```python
from build123d import *

# Parameters (mm, degrees)
F1_DEPTH = 40
F0_W     = 0.5
F0_H     = 12
F0_W_2   = 11.5
F0_W_3   = 12
F0_H_2   = 0.5
F0_H_3   = 14.25
F2_DEPTH = 5
F3_SIZE  = 2
F5_DEPTH = 0.5


with BuildPart() as f1:
    # F0 (on Top) → F1 (new body)
    with BuildSketch(Plane.XY):
        Polygon((17.2627416998, 5.4343145751), (15, 3.1715728753), (15, -3.1715728753), (17.2627416998, -5.4343145751), (17.2627416998, -0.5656854249), (17.2627416998, 0.5656854249), align=None)
        Polygon((-15, 29.1715728753), (-15, 4.1715728753), (-12.1715728752, 7), (-12.1715728752, 0), (-12.1715728752, -7), (-15, -4.1715728753), (-15, -29.1715728753), (15, -29.1715728753), (15, -3.1715728753), (15, 3.1715728753), (15, 29.1715728753), align=None)
        Polygon((-10.4999961331, 14.999999851), (-10.4999961331, 26.999999851), (1.5000038669, 26.999999851), (2.0000038669, 26.999999851), (13.5000038669, 26.999999851), (13.5000038669, 14.999999851), (13.5000038669, 14.499999851), (13.5000038669, 0.249999851), (13.5000038669, -0.250000149), (13.5000038669, -14.500000149), (13.5000038669, -15.000000149), (13.5000038669, -27.000000149), (2.0000038669, -27.000000149), (1.5000038669, -27.000000149), (-10.4999961331, -27.000000149), (-10.4999961331, -15.000000149), (-10.4999961331, -14.500000149), (-10.4999961331, -0.250000149), (-10.4999961331, 0.249999851), (-10.4999961331, 14.499999851), align=None, mode=Mode.SUBTRACT)
    extrude(amount=F1_DEPTH)

    # F0 (on Top) → F2 (join)
    with BuildSketch(Plane.XY):
        Polygon((-15, 29.1715728753), (-15, 4.1715728753), (-12.1715728752, 7), (-12.1715728752, 0), (-12.1715728752, -7), (-15, -4.1715728753), (-15, -29.1715728753), (15, -29.1715728753), (15, -3.1715728753), (15, 3.1715728753), (15, 29.1715728753), align=None)
        Polygon((-10.4999961331, 14.999999851), (-10.4999961331, 26.999999851), (1.5000038669, 26.999999851), (2.0000038669, 26.999999851), (13.5000038669, 26.999999851), (13.5000038669, 14.999999851), (13.5000038669, 14.499999851), (13.5000038669, 0.249999851), (13.5000038669, -0.250000149), (13.5000038669, -14.500000149), (13.5000038669, -15.000000149), (13.5000038669, -27.000000149), (2.0000038669, -27.000000149), (1.5000038669, -27.000000149), (-10.4999961331, -27.000000149), (-10.4999961331, -15.000000149), (-10.4999961331, -14.500000149), (-10.4999961331, -0.250000149), (-10.4999961331, 0.249999851), (-10.4999961331, 14.499999851), align=None, mode=Mode.SUBTRACT)
        Polygon((-12.1715728752, 7), (-15, 4.1715728753), (-15, -4.1715728753), (-12.1715728752, -7), (-12.1715728752, 0), align=None)
        with Locations((1.7500038669, -21.000000149)):
            Rectangle(F0_W, F0_H)
        with Locations((7.7500038669, -21.000000149)):
            Rectangle(F0_W_2, F0_H)
        with Locations((-4.4999961331, -21.000000149)):
            Rectangle(F0_W_3, F0_H)
        with Locations((-4.4999961331, -14.750000149)):
            Rectangle(F0_W_3, F0_H_2)
        with Locations((1.7500038669, -14.750000149)):
            Rectangle(F0_W, F0_H_2)
        with Locations((1.7500038669, -7.375000149)):
            Rectangle(F0_W, F0_H_3)
        with Locations((-4.4999961331, -7.375000149)):
            Rectangle(F0_W_3, F0_H_3)
        with Locations((7.7500038669, -7.375000149)):
            Rectangle(F0_W_2, F0_H_3)
        with Locations((7.7500038669, 7.374999851)):
            Rectangle(F0_W_2, F0_H_3)
        with Locations((-4.4999961331, 7.374999851)):
            Rectangle(F0_W_3, F0_H_3)
        with Locations((1.7500038669, -1.49e-07)):
            Rectangle(F0_W, F0_H_2)
        with Locations((1.7500038669, 7.374999851)):
            Rectangle(F0_W, F0_H_3)
        with Locations((7.7500038669, 14.749999851)):
            Rectangle(F0_W_2, F0_H_2)
        with Locations((1.7500038669, 14.749999851)):
            Rectangle(F0_W, F0_H_2)
        with Locations((-4.4999961331, 14.749999851)):
            Rectangle(F0_W_3, F0_H_2)
        with Locations((-4.4999961331, 20.999999851)):
            Rectangle(F0_W_3, F0_H)
        with Locations((7.7500038669, 20.999999851)):
            Rectangle(F0_W_2, F0_H)
        with Locations((1.7500038669, 20.999999851)):
            Rectangle(F0_W, F0_H)
        with Locations((-4.4999961331, -1.49e-07)):
            Rectangle(F0_W_3, F0_H_2)
        with Locations((7.7500038669, -1.49e-07)):
            Rectangle(F0_W_2, F0_H_2)
        with Locations((7.7500038669, -14.750000149)):
            Rectangle(F0_W_2, F0_H_2)
    extrude(amount=-F2_DEPTH)

    # F3
    f3_edges = [f1.edges().sort_by_distance(p)[0] for p in [
        (0, -29.171573, -5),
        (0, 29.171573, -5),
        (0, -29.171573, 40),
        (0, 29.171573, 40),
    ]]
    chamfer(f3_edges, length=F3_SIZE)

    # F4 (on face) → F5 (cut)
    with BuildSketch(Plane(origin=(-12.1715728752, 0, 0), x_dir=(0, -1, 0), z_dir=(-1, 0, 0))):
        with BuildLine():
            Line((0.12, 10.25), (0.12, 10.5))
            ThreePointArc((0.12, 10.5), (-1.8790989856, 8.5600270426), (0, 6.5036032458))
            Line((0, 6.5036032458), (0, 6.7541191335))
            ThreePointArc((0, 6.7541191335), (-1.6289699135, 8.5600353381), (0.12, 10.25))
        make_face()
        with BuildLine():
            Line((0, 8.5), (0, 6.7541191335))
            ThreePointArc((0, 6.7541191335), (0.1250128042, 6.7500071795), (0.25, 6.7548352513))
            Line((0.25, 6.7548352513), (0.25, 8.25))
            Line((0.25, 8.25), (1.8520508076, 8.25))
            ThreePointArc((1.8520508076, 8.25), (1.865506934, 8.3746782406), (1.87, 8.5))
            Line((1.87, 8.5), (0, 8.5))
        make_face()
        with BuildLine():
            Line((0.25, 6.7548352513), (0.25, 6.5042294721))
            ThreePointArc((0.25, 6.5042294721), (1.5794519519, 7.1325205669), (2.12, 8.5))
            Line((2.12, 8.5), (1.87, 8.5))
            ThreePointArc((1.87, 8.5), (1.865506934, 8.3746782406), (1.8520508076, 8.25))
            ThreePointArc((1.8520508076, 8.25), (1.3140216535, 7.2206203491), (0.25, 6.7548352513))
        make_face()
        with BuildLine():
            Line((0, 6.7541191335), (0, 6.5036032458))
            ThreePointArc((0, 6.5036032458), (0.1250097944, 6.5000062745), (0.25, 6.5042294721))
            Line((0.25, 6.5042294721), (0.25, 6.7548352513))
            ThreePointArc((0.25, 6.7548352513), (0.1250128042, 6.7500071795), (0, 6.7541191335))
        make_face()
        with BuildLine():
            ThreePointArc((0.25, 6.5042294721), (0.1250097944, 6.5000062745), (0, 6.5036032458))
            Line((0, 6.5036032458), (0, 5))
            Line((0, 5), (0.25, 5))
            Line((0.25, 5), (0.25, 6.5042294721))
        make_face()
    extrude(amount=-F5_DEPTH, mode=Mode.SUBTRACT)


solid = f1.part
```
Geometry check sheet. Reference: the model listing, model coordinates, mm. A direction names the side the tool comes from. Give positions to 0.01 mm unless a question says otherwise; leave off trailing zeros. Order: outer loops, then holes, each group sorted by start corner. A loop starts at its lowest first (then second) coordinate and runs counter-clockwise, first axis right, second up. Notation, with made-up numbers: (56, -37.5) - (112, -37.5) arc R13 cw to (112, -31.5) - close; hole circle Ø10 at (-31.75, -3). An arc over 180 degrees is marked (long way). Answer in a Markdown table with one row per item. Add a question column.
Q1. Mould release check, pull along X, two halves, no side actions. Record for faces 1 (the flat face through (-15, 7, 18)), 2 (the flat face through (-11, 0, 40)), 3 (the flat face through (-13.606, 5.566, 19.72)): pulls with the +X half, pulls with the -X half, needs draft (parallel to the pull), parting line crosses it, or undercut.
Q2. Tool access check on faces 4 (the cylindrical face through (-11.93, 1.63, 8.52)), 5 (the flat face through (16, 0, 0)), 6 (the flat face through (-14, 0, 0)), 7 (the flat face through (0, 29.172, 18)). Record the directions out of +Z, -Z, +X, -X, +Y, -Y that give a thin tool (end or side, any length) a straight path to the whole face; none if there is none.
Q3. Cross-section at A-A, the plane z = 11.5. Enter the section's corners in (x, y).
Q4. Cross-section at B-B, the plane x = 10. Enter the section's corners in (y, z).
Q5. Cross-section at C-C, the plane y = 18.5. Enter the section's corners in (x, z).
Q6. Gauge pin test, flat ends, axial feed: pin 1 (2 mm diameter, centred on y = 0, z = 7, fed in from -X); pin 2 (20 mm diameter, centred on y = -2, z = 13.5, fed in from -X); pin 3 (8 mm diameter, centred on x = 7, y = -10, fed in from +Z); pin 4 (1.5 mm diameter, centred on y = -21, z = 17, fed in from +X). Record the tip position at first contact, or that the pin passes through.
Q7. Material ranges on probe 1 along Y at (x, z) = (5, 16.5); probe 2 along X at (y, z) = (-4.5, 4); probe 3 along X at (y, z) = (8.5, 31), recorded low to high. Write a range as from..to.
Check values:
| question | item | result |
|---|---|---|
| 1 | face 1 | pulls with the -X half |
| 1 | face 2 | needs draft |
| 1 | face 3 | undercut |
| 2 | face 4 | -X |
| 2 | face 5 | -Z, +X, +Y, -Y |
| 2 | face 6 | +Z |
| 2 | face 7 | +Z, -Z, +X, -X, +Y |
| 3 | outline | (-15, -29.17) - (15, -29.17) - (15, -3.17) - (17.26, -5.43) - (17.26, 5.43) - (15, 3.17) - (15, 29.17) - (-15, 29.17) - (-15, 4.17) - (-12.17, 7) - (-12.17, -7) - (-15, -4.17) - close; hole (-10.5, -27) - (13.5, -27) - (13.5, 27) - (-10.5, 27) - close |
| 4 | outline | (-29.17, -3) - (-27.17, -5) - (27.17, -5) - (29.17, -3) - (29.17, 38) - (27.17, 40) - (27, 40) - (27, 0) - (-27, 0) - (-27, 40) - (-27.17, 40) - (-29.17, 38) - close |
| 5 | outline | (-15, -5) - (15, -5) - (15, 40) - (13.5, 40) - (13.5, 0) - (-10.5, 0) - (-10.5, 40) - (-15, 40) - close |
| 6 | pin 1 | stops at x = -12.17 |
| 6 | pin 2 | stops at x = -15 |
| 6 | pin 3 | stops at z = 0 |
| 6 | pin 4 | stops at x = 15 |
| 7 | probe 1 | y = -29.17..-27, 27..29.17 |
| 7 | probe 2 | x = -15..-14.67, -12.17..-10.5, 13.5..15, 16.33..17.26 |
| 7 | probe 3 | x = -15..-10.5, 13.5..15 |
